from build123d import *

# Parameters (mm, degrees)
BOSS_EXTRUDE1_DEPTH = 25.4


with BuildPart() as part:
    # Sketch1 → Boss-Extrude1 (new body)
    with BuildSketch(Plane.XY):
        with BuildLine():
            Line((0, 0), (8.443048692, 0))
            Line((8.443048692, 0), (8.443048692, -2.2352))
            Line((8.443048692, -2.2352), (4.201248692, -2.2352))
            Line((4.201248692, -2.2352), (9.878148692, -6.315260883))
            Line((9.878148692, -6.315260883), (12.849948692, -6.315260883))
            Line((12.849948692, -6.315260883), (18.526848692, -2.2352))
            Line((18.526848692, -2.2352), (14.285048692, -2.2352))
            Line((14.285048692, -2.2352), (14.285048692, 0))
            Line((14.285048692, 0), (25.4, 0))
            Line((25.4, 0), (25.4, 9.829452055))
            Line((25.4, 9.829452055), (17.484246575, 9.829452055))
            ThreePointArc((17.484246575, 9.829452055), (12.7, 5.045205479), (7.915753425, 9.829452055))
            Line((7.915753425, 9.829452055), (0, 9.829452055))
            Line((0, 9.829452055), (0, 0))
        make_face()
    extrude(amount=BOSS_EXTRUDE1_DEPTH)


solid = part.part
Model file for the job. Use its own axes, mm. A direction names the side the tool comes from. Give positions to 0.01 mm unless a question says otherwise; leave off trailing zeros. Order: outer loops, then holes, each group sorted by start corner. A loop starts at its lowest first (then second) coordinate and runs counter-clockwise, first axis right, second up. Notation, with made-up numbers: (62, 88.5) - (77, 88.5) arc R22 ccw to (77, 104.5) - close; hole circle Ø7 at (66.5, 38). An arc over 180 degrees is marked (long way). Return JSON: item names as keys, results as strings.
1) 3-axis set-ups, long thin cutter, end or side, ignore diameter. For faces 4 (the flat face through (13, 4, 0)), 5 (the flat face through (14.285, -1, 13)), 6 (the flat face through (8.443, -1, 13)): which of +Z, -Z, +X, -X, +Y, -Y reach the whole face in a straight line?
Geometry says:
{"face 4": "-Z, +X, -X, +Y, -Y", "face 5": "+Z, -Z, +X", "face 6": "+Z, -Z, -X"}
2) Flat gauge pins, fed straight in: P1, Ø2.5, axis at y = -1.5, z = 11.5, coming from the +X side; P2, Ø2, axis at x = 5.5, z = 4.5, coming from the -Y side; P3, Ø5, axis at x = 5, z = 6, coming from the -Y side. Where does each tip first touch, or does it go through?
Geometry says:
{"P1": "x = 18.53", "P2": "y = -3.89", "P3": "y = -4.61"}
3) Cut at B-B, the plane z = 12. Give the cut face in (x, y).
Geometry says:
{"outline": "(0, 0) - (8.44, 0) - (8.44, -2.24) - (4.2, -2.24) - (9.88, -6.32) - (12.85, -6.32) - (18.53, -2.24) - (14.29, -2.24) - (14.29, 0) - (25.4, 0) - (25.4, 9.83) - (17.48, 9.83) arc R4.78 cw to (7.92, 9.83) - (0, 9.83) - close"}
4) Pull direction Y, two halves, no side cores. Call faces 1 (the flat face through (0, 5, 13)), 2 (the flat face through (21, 9.829, 13)), 3 (the flat face through (16, -2.235, 13)): pulls with the +Y half, pulls with the -Y half, needs draft (parallel to the pull), parting line crosses it, or undercut.
Geometry says:
{"face 1": "needs draft", "face 2": "pulls with the +Y half", "face 3": "undercut"}
5) Cut at A-A, the plane x = 17. Give the cut face in (y, z).
Geometry says:
{"outline": "(-3.33, 0) - (-2.24, 0) - (-2.24, 25.4) - (-3.33, 25.4) - close; (0, 0) - (7.73, 0) - (7.73, 25.4) - (0, 25.4) - close"}
6) Cut at C-C, the plane x = 23.25. Give the cut face in (y, z).
Geometry says:
{"outline": "(0, 0) - (9.83, 0) - (9.83, 25.4) - (0, 25.4) - close"}
7) Cut at D-D, the plane y = -1.25. Give the cut face in (x, z).
Geometry says:
{"outline": "(8.44, 0) - (14.29, 0) - (14.29, 25.4) - (8.44, 25.4) - close"}
8) Probe line 1 (Y direction, x = 12.75, z = 1.5); line 2 (Y direction, x = 24, z = 18); line 3 (Y direction, x = 16.75, z = 13.25). List the from-to ranges inside material, lowest first. Write a range as from..to.
Geometry says:
{"line 1": "-6.32..5.05", "line 2": "0..9.83", "line 3": "-3.51..-2.24, 0..7.28"}
